```python
from build123d import *

# Parameters (mm, degrees)
BOSS_EXTRUDE1_DEPTH = 4.826
SKETCH2_W           = 25.4
SKETCH2_H           = 4.826
CUT_EXTRUDE1_DEPTH  = 4.826


with BuildPart() as part:
    # Sketch1 → Boss-Extrude1 (new body)
    with BuildSketch(Plane.XY):
        Polygon((95.25, 50.8), (95.25, 25.4), (90.424, 25.4), (90.424, 0), (95.25, 0), (527.05, 0), (531.876, 0), (531.876, 25.4), (527.05, 25.4), (527.05, 50.8), (531.876, 50.8), (531.876, 76.2), (527.05, 76.2), (527.05, 101.6), (531.876, 101.6), (531.876, 127), (90.424, 127), (90.424, 101.6), (95.25, 101.6), (95.25, 76.2), (90.424, 76.2), (90.424, 50.8), align=None)
    extrude(amount=BOSS_EXTRUDE1_DEPTH)

    # Sketch2 → Cut-Extrude1 (cut)
    with BuildSketch(Plane(origin=(0, 127, 0), x_dir=(1, 0, 0), z_dir=(0, 1, 0))):
        with Locations((133.35, -2.413)):
            Rectangle(SKETCH2_W, SKETCH2_H)
        with Locations((184.15, -2.413)):
            Rectangle(SKETCH2_W, SKETCH2_H)
        with Locations((234.95, -2.413)):
            Rectangle(SKETCH2_W, SKETCH2_H)
        with Locations((285.75, -2.413)):
            Rectangle(SKETCH2_W, SKETCH2_H)
        with Locations((336.55, -2.413)):
            Rectangle(SKETCH2_W, SKETCH2_H)
        with Locations((387.35, -2.413)):
            Rectangle(SKETCH2_W, SKETCH2_H)
        with Locations((438.15, -2.413)):
            Rectangle(SKETCH2_W, SKETCH2_H)
        with Locations((488.95, -2.413)):
            Rectangle(SKETCH2_W, SKETCH2_H)
    extrude(amount=-CUT_EXTRUDE1_DEPTH, mode=Mode.SUBTRACT)


solid = part.part
```
Input: part model. Units: mm. Frame: model coordinates. Give positions to 0.01 mm unless a question says otherwise; leave off trailing zeros. Order: outer loops, then holes, each group sorted by start corner. A loop starts at its lowest first (then second) coordinate and runs counter-clockwise, first axis right, second up. Notation, with made-up numbers: M 41,62.5 L 47,62.5 A20 ccw 47,90.5 Z; hole C -24.5,-35.5 d4. An arc over 180 degrees is marked long. Return JSON: item names as keys, results as strings.
1) Section query A-A on y = 40. Output: boundary loops of the cut face in (x, z).
Taken from the geometry:
{"outline": "M 95.25,0 L 527.05,0 L 527.05,4.83 L 95.25,4.83 Z"}
2) Section query B-B on x = 241. Output: boundary loops of the cut face in (y, z), and give its area (3 significant figures).
Taken from the geometry:
{"outline": "M 0,0 L 122.17,0 L 122.17,4.83 L 0,4.83 Z", "area": "590 mm2"}
3) Line query: L1, parallel to Y at x = 343, z = 1.9; L2, parallel to X at y = 99.5, z = 4.5. Output: solid intervals per line, ascending. Write a range as [from, to].
Taken from the geometry:
{"L1": "y = [0, 122.17]", "L2": "x = [95.25, 527.05]"}
4) Contact query for a flat-ended pin moving along its axis: pin 1 (1.4 mm diameter, centred on x = 332, z = 2.5, fed in from +Y). Output: stop coordinate, or through.
Taken from the geometry:
{"pin 1": "stops at y = 122.17"}
